```python
from build123d import *

# Parameters (mm, degrees)
F0_W     = 50.8
F0_H     = 50.8
F1_DEPTH = 38.1
F2_R     = 0.635
F3_DEPTH = 1.27
F5_DEPTH = 50.801
F6_R     = 2.54


with BuildPart() as f1:
    # F0 (on Top) → F1 (new body, symmetric)
    with BuildSketch(Plane.XY):
        Rectangle(F0_W, F0_H)
    extrude(amount=F1_DEPTH, both=True)

    # F2 (on face) → F3 (cut)
    with BuildSketch(Plane.XY.offset(38.1)):
        with Locations((-7.62, 0)):
            Circle(F2_R)
        with Locations((7.62, 0)):
            Circle(F2_R)
    extrude(amount=-F3_DEPTH, mode=Mode.SUBTRACT)

    # F4 (on face) → F5 (cut, through all)
    with BuildSketch(Plane.YZ.offset(25.4)):
        Polygon((-25.4, 38.1), (-25.4, 20.32), (-7.62, 38.1), align=None)
    extrude(amount=-F5_DEPTH, mode=Mode.SUBTRACT)

    # F6
    f6_edges = [f1.edges().sort_by_distance(p)[0] for p in [
        (0, -7.62, 38.1),
        (0, -25.4, 20.32),
        (25.4, -16.51, 29.21),
        (25.4, 8.89, 38.1),
        (0, 25.4, 38.1),
        (25.4, 25.4, 0),
        (-25.4, 8.89, 38.1),
        (-25.4, -16.51, 29.21),
        (25.4, -25.4, -8.89),
        (-25.4, -25.4, -8.89),
        (-25.4, 25.4, 0),
    ]]
    fillet(f6_edges, radius=F6_R)


solid = f1.part
```
The model under review builds one solid part; all positions refer to its coordinate system, in mm. Round coordinates to 2 decimals unless told otherwise and drop trailing zeros. Write each loop counter-clockwise with the first axis right and the second up, starting at its lowest first coordinate (ties: lowest second). Pieces come first, ordered by that corner, then holes. Notation, with made-up numbers: (-21.5, 58.25) - (5.5, 58.25) arc R14 ccw to (5.5, 76.25) - close; hole circle Ø10 at (31, 15). An arc over 180 degrees is marked (long way). Answer as CSV lines item,"result". Start each with the question number.
(1) For pin 1 Ø1 at (x, y) = (-7.62, 0) entering from +Z, flat-tipped, find the tip position at first contact; note if it passes through.
(2) To check wall thickness, follow line 1 (Y direction, x = 7.62, z = 37.75) (3 decimals); line 2 (Z direction, x = -3.5, y = 23); line 3 (Z direction, x = -23, y = -7.5). State the ranges of each line that lie inside material, in increasing order.
(3) We need section A-A on x = -15. State the section outline as (y, z) points.
Worked answers:
1,pin 1,"z = 36.83"
2,line 1,"-7.855 to -0.635, 0.635 to 24.147"
2,line 2,"-38.1 to 38.1"
2,line 3,"-38.1 to 37.92"
3,outline,"(-25.4, -38.1) - (25.4, -38.1) - (25.4, 35.56) arc R2.54 ccw to (22.86, 38.1) - (-6.57, 38.1) arc R2.54 ccw to (-8.36, 37.36) - (-24.66, 21.06) arc R2.54 ccw to (-25.4, 19.27) - close"
